Could you check a few things on this drawing? It's one solid part, dimensions in mm from its lowest x, y, z. Coordinates: 2 decimals unless noted, no trailing zeros. Loops run counter-clockwise (first coordinate to the right, second up) from the corner with the lowest first, then second, coordinate; pieces in that order, holes last. Notation, with made-up numbers: M -29,81.25 L 5,81.25 A8 cw 5,91.25 Z; hole C 53.5,67 d3. An arc over 180 degrees is marked long. Use one line per item in the form item = value. Start each with the question number.
(1) Imagine slicing it at A-A, the plane z = 6.25. Please give me the cut outline in (x, y).
(2) Imagine slicing it at B-B, the plane y = 32.5. Please give me the cut outline in (x, z).
(3) Imagine slicing it at C-C, the plane x = 227. Please give me the cut outline in (y, z).
(4) Please list where these lines run through material, in increasing order: L1, parallel to X at y = 125.5, z = 2; L2, parallel to Y at x = 147, z = 7.25; L3, parallel to Y at x = 205.5, z = 1.25.
(5) Will these pins go through, and if not, where does the flat tip stop? P1, Ø1, axis at y = 143.5, z = 1.5, coming from the -X side; P2, Ø5, axis at x = 3.5, z = 3, coming from the +Y side; P3, Ø2, axis at x = 145.5, z = 2.5, coming from the -Y side.
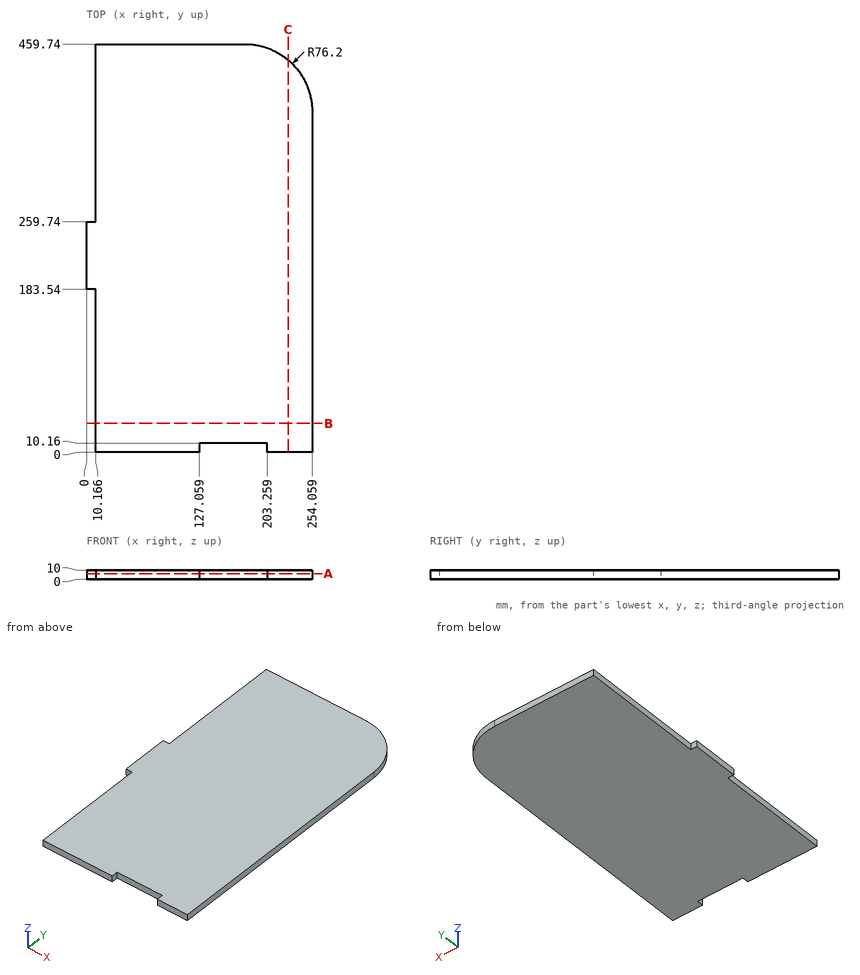
Answer:
q1.outline = M 0,183.54 L 10.17,183.54 L 10.17,0 L 127.06,0 L 127.06,10.16 L 203.26,10.16 L 203.26,0 L 254.06,0 L 254.06,383.54 A76.2 ccw 177.86,459.74 L 10.17,459.74 L 10.17,259.74 L 0,259.74 Z
q2.outline = M 10.17,0 L 254.06,0 L 254.06,10 L 10.17,10 Z
q3.outline = M 0,0 L 441.78,0 L 441.78,10 L 0,10 Z
q4.L1 = 10.17 to 254.06
q4.L2 = 10.16 to 459.74
q4.L3 = 0 to 454.55
q5.P1 = 10.17
q5.P2 = 259.74
q5.P3 = 10.16
